Autodesk Inventor part; units mm, degrees
ref_plane "YZ Plane" through (0, 0, 0) normal (1, 0, 0) x (0, 1, 0)
ref_plane "XZ Plane" through (0, 0, 0) normal (0, 1, 0) x (-1, 0, 0)
ref_plane "XY Plane" through (0, 0, 0) normal (0, 0, 1) x (1, 0, 0)
sketch "草圖1" plane through (0, 0, 0) normal (0, 1, 0) x (-1, 0, 0)
  circle A0 centre (0, 0) radius 70
  circle A1 centre (0, 0) radius 25
  line L0 (-70, 10) -> (-10, 10)
  line L1 (-10, 10) -> (-10, -10)
  line L2 (-10, -10) -> (-70, -10)
  line L3 (-70, -10) -> (-70, 10)
  line L4 (0, 0) -> (0, -55)
  line L5 (0, 0) -> (35.3533, -42.1324)
  arc A2 (0, -55) -> (35.3533, -42.1324) centre (0, 0) ccw
  line L6 (0, 0) -> (51.6831, -18.8111)
  line L7 (0, 0) -> (51.6831, 18.8111)
  arc A3 (51.6831, -18.8111) -> (51.6831, 18.8111) centre (0, 0) ccw
  line L8 (0, 0) -> (35.3533, 42.1324)
  line L9 (0, 0) -> (0, 55)
  arc A4 (35.3533, 42.1324) -> (0, 55) centre (0, 0) ccw
  line L10 (-9.3, -13.3795) -> (-36.7, -13.3795)
  line L11 (-36.7, -13.3795) -> (-36.7, -69.3795)
  line L12 (-36.7, -69.3795) -> (-9.3, -69.3795)
  line L13 (-9.3, -69.3795) -> (-9.3, -13.3795)
  line L14 (-7.8, -20.3795) -> (-10.8, -20.3795)
  line L15 (-10.8, -20.3795) -> (-10.8, -27.3795)
  line L16 (-10.8, -27.3795) -> (-7.8, -27.3795)
  line L17 (-7.8, -27.3795) -> (-7.8, -20.3795)
  line L18 (-7.8, -55.3795) -> (-10.8, -55.3795)
  line L19 (-10.8, -55.3795) -> (-10.8, -62.3795)
  line L20 (-10.8, -62.3795) -> (-7.8, -62.3795)
  line L21 (-7.8, -62.3795) -> (-7.8, -55.3795)
  line L22 (-35.2, -20.3795) -> (-38.2, -20.3795)
  line L23 (-38.2, -20.3795) -> (-38.2, -27.3795)
  line L24 (-38.2, -27.3795) -> (-35.2, -27.3795)
  line L25 (-35.2, -27.3795) -> (-35.2, -20.3795)
  line L26 (-35.2, -48.3795) -> (-38.2, -48.3795)
  line L27 (-38.2, -48.3795) -> (-38.2, -55.3795)
  line L28 (-38.2, -55.3795) -> (-35.2, -55.3795)
  line L29 (-35.2, -55.3795) -> (-35.2, -48.3795)
  circle A5 centre (0, 0) radius 2
  line L30 (-1.5, 1.3229) -> (-1.5, -1.3229)
  point P0 (-23, -13.3795)
  point P1 (-9.3, -20.3795)
  point P2 (-9.3, -62.3795)
  point P3 (-36.7, -20.3795)
  point P4 (-36.7, -48.3795)
  point P5 (16.0697, -19.1511)
  point P6 (0, -25)
  point P7 (-69.282, 10)
  point P8 (-69.282, -10)
  point P9 (16.0697, 19.1511)
  point P10 (0, 25)
  point P11 (23.4923, -8.5505)
  point P12 (23.4923, 8.5505)
  point P13 (-70, 0)
  dimension "d0" = 140
  dimension "d1" = 50
  dimension "d2" = 20
  dimension "d3" = 60
  dimension "d4" = 55
  dimension "d5" = 40
  dimension "d6" = 55
  dimension "d9" = 140
  dimension "d11" = 13
  dimension "d12" = 27.4
  dimension "d13" = 56
  dimension "d14" = 7
  dimension "d15" = 3
  dimension "d16" = 7
  dimension "d17" = 7
  dimension "d18" = 3
  dimension "d19" = 7
  dimension "d20" = 7
  dimension "d21" = 3
  dimension "d22" = 7
  dimension "d23" = 7
  dimension "d24" = 3
  dimension "d25" = 21
  dimension "d28" = 4
  dimension "d29" = 1.5
extrude "擠出1" add sketch "草圖1" along normal blind 3 contours L13 L20 L21 L18 L16 L17 A1 L4 A2 L5 L6 A3 L7 L8 A4 L9 L0 A0 | A0 L11 L28 L29 L26 L24 L25 L22 L10 A1 L15 L16 L13 L18 L19 L20 | A0 L2 A1 L10 L11 L22 L23 L24 L26 L27 L28 | L20 L19 L18 L13 | L13 L18 L21 L20 | L28 L27 L26 L11 | L11 L26 L29 L28 | A1 L9 A5 L4 L17 L14 L13 L10 L2 L1 L0 | L16 L15 A1 L13 | L13 A1 L17 L16 | A1 L8 A5 L9 | L10 L13 L14 L15 A1 | L24 L23 L22 L11 | L11 L22 L25 L24 | L13 L14 L17 A1 | A1 L15 L14 L13 | A1 L7 A5 L8 | A1 L6 A5 L7 | L30 A5 | L4 A5 L5 A1 | A5 L6 A1 L5
sketch "草圖2" plane through (0, 3, 0) normal (0, 1, 0) x (1, 0, 0)
  line L0 (-66, 3) -> (-63, 3)
  line L1 (-63, 3) -> (-63, -3)
  line L2 (-63, -3) -> (-66, -3)
  line L3 (-66, -3) -> (-66, 3)
  line L4 (-35.5981, -55.6577) -> (-34.0981, -53.0596)
  line L5 (-34.0981, -53.0596) -> (-28.9019, -56.0596)
  line L6 (-28.9019, -56.0596) -> (-30.4019, -58.6577)
  line L7 (-30.4019, -58.6577) -> (-35.5981, -55.6577)
  line L8 (30.4019, -58.6577) -> (28.9019, -56.0596)
  line L9 (28.9019, -56.0596) -> (34.0981, -53.0596)
  line L10 (34.0981, -53.0596) -> (35.5981, -55.6577)
  line L11 (35.5981, -55.6577) -> (30.4019, -58.6577)
  line L12 (66, -3) -> (63, -3)
  line L13 (63, -3) -> (63, 3)
  line L14 (63, 3) -> (66, 3)
  line L15 (66, 3) -> (66, -3)
  line L16 (35.5981, 55.6577) -> (34.0981, 53.0596)
  line L17 (34.0981, 53.0596) -> (28.9019, 56.0596)
  line L18 (28.9019, 56.0596) -> (30.4019, 58.6577)
  line L19 (30.4019, 58.6577) -> (35.5981, 55.6577)
  line L20 (-30.4019, 58.6577) -> (-28.9019, 56.0596)
  line L21 (-28.9019, 56.0596) -> (-34.0981, 53.0596)
  line L22 (-34.0981, 53.0596) -> (-35.5981, 55.6577)
  line L23 (-35.5981, 55.6577) -> (-30.4019, 58.6577)
  point P0 (0, 0)
  point P1 (-63, 0)
  point P2 (-31.5, -54.5596)
  point P3 (31.5, -54.5596)
  point P4 (63, 0)
  point P5 (31.5, 54.5596)
  point P6 (-31.5, 54.5596)
  dimension "d30" = 3
  dimension "d31" = 6
  dimension "d32" = 63
  dimension "d37" = 360
extrude "擠出2" cut sketch "草圖2" against normal through all contours L0 L1 L2 L3 | L4 L5 L6 L7 | L8 L9 L10 L11 | L16 L17 L18 L19 | L20 L21 L22 L23
sketch "草圖3" plane through (0, 3, 0) normal (0, 1, 0) x (1, 0, 0)
  line L0 (-3, 13) -> (3, 13)
  line L1 (3, 13) -> (3, 10)
  line L2 (3, 10) -> (-3, 10)
  line L3 (-3, 10) -> (-3, 13)
  line L4 (-12.7583, 3.9019) -> (-9.7583, 9.0981)
  line L5 (-9.7583, 9.0981) -> (-7.1603, 7.5981)
  line L6 (-7.1603, 7.5981) -> (-10.1603, 2.4019)
  line L7 (-10.1603, 2.4019) -> (-12.7583, 3.9019)
  line L8 (-9.7583, -9.0981) -> (-12.7583, -3.9019)
  line L9 (-12.7583, -3.9019) -> (-10.1603, -2.4019)
  line L10 (-10.1603, -2.4019) -> (-7.1603, -7.5981)
  line L11 (-7.1603, -7.5981) -> (-9.7583, -9.0981)
  line L12 (3, -13) -> (-3, -13)
  line L13 (-3, -13) -> (-3, -10)
  line L14 (-3, -10) -> (3, -10)
  line L15 (3, -10) -> (3, -13)
  point P0 (0, 0)
  point P1 (0, 10)
  point P2 (-8.6603, 5)
  point P3 (-8.6603, -5)
  point P4 (0, -10)
  dimension "d39" = 6
  dimension "d40" = 3
  dimension "d41" = 10
  dimension "d44" = 180
extrude "擠出3" cut sketch "草圖3" against normal through all
properties part number "rolling_plate"
The listing builds one solid part. Answer for the finished solid, in the listing's coordinates (mm). Round coordinates to 2 decimals unless told otherwise and drop trailing zeros. Write each loop counter-clockwise with the first axis right and the second up, starting at its lowest first coordinate (ties: lowest second). Pieces come first, ordered by that corner, then holes. Notation, with made-up numbers: (0.5, 28) -> (23.5, 28) arc R13 cw to (23.5, 42) -> close; hole circle Ø10 at (-14.5, 67). An arc over 180 degrees is marked (long way). Write item = value, one per line.
1) Straight lines are drawn through the part: line 1 along X through (y, z) = (0.95, 0); line 2 along X through (y, z) = (1.3, -57); line 3 along Z through (x, y) = (-27, 2.65). For each, find the intervals that lie inside material, in ascending order. Write a range as [from, to].
Check values:
line_1 = [-70, -66], [-63, -55], [-25, -2], [1.5, 10]
line_2 = [-40.63, -33.27], [-29.44, 29.44], [33.27, 40.63]
line_3 = [-64.58, -47.92], [-32.18, -9.83], [9.83, 32.18], [47.92, 64.58]
2) Section B-B on z = 49 is taken. Write down the section's boundary in (x, y), plus the area to 3 significant figures.
Check values:
outline = (-49.99, 0) -> (-24.98, 0) -> (-24.98, 3) -> (-49.99, 3) -> close; (0, 0) -> (49.99, 0) -> (49.99, 3) -> (0, 3) -> close
area = 225 mm²
3) For a pull along Z with two mould halves and no side action, classify faces 1 (the flat face through (1, 0, -15)), 2 (the cylindrical face through (-18.558, 1.479, 51.774)) as released by +Z, released by -Z, zero draft, split by the parting line, or undercut.
Check values:
face_1 = zero draft
face_2 = undercut
4) Section C-C on y = 0.85 is taken. Give the number of separate pieces and of enclosed holes in the cut face, plus the area to 3 significant figures.
Check values:
separate_pieces = 1
enclosed_holes = 13
area = 11,500 mm²
5) Section A-A on x = 58.5 is taken. Write down the section's boundary in (y, z), plus the area to 3 significant figures.
Check values:
outline = (0, -38.44) -> (3, -38.44) -> (3, -10) -> (0, -10) -> close; (0, 10) -> (3, 10) -> (3, 38.44) -> (0, 38.44) -> close
area = 171 mm²
6) Section D-D on x = -58 is taken. Write down the section's boundary in (y, z), plus the area to 3 significant figures.
Check values:
outline = (0, -39.19) -> (3, -39.19) -> (3, 39.19) -> (0, 39.19) -> close
area = 235 mm²
7) Given pin 1 (1.5 mm diameter, centred on y = 1, z = -4.5, fed in from -X); pin 2 (0.9 mm diameter, centred on x = -64.5, y = 1.5, fed in from +Z); pin 3 (0.9 mm diameter, centred on y = 1, z = -11.5, fed in from +X), each flat-ended and moving along its own axis, determine where each tip first touches the part or whether it passes through.
Check values:
pin_1 = -69.9
pin_2 = 28.24
pin_3 = 69.12
